Here's the drawing with two shaded views (mm, measured from the low corner). I have some questions. A direction names the side the tool comes from. Round coordinates to 2 decimals unless told otherwise and drop trailing zeros. Loops run counter-clockwise (first coordinate to the right, second up) from the corner with the lowest first, then second, coordinate; pieces in that order, holes last.
(1) I want a section at D-D on y = 43. Write out the boundary of the cut face in (x, z).
(2) Thinking about a two-plate mould opening in X: for the marked faces 4, 5 and 6, which applies, released by +X, released by -X, zero draft, split by the parting line, or undercut?
(3) Will these pins go through, and if not, where does the flat tip stop? pin 1 Ø12 at (x, z) = (18.5, 36.5) entering from +Y; pin 2 Ø1 at (x, z) = (39, 53.5) entering from -Y; pin 3 Ø6 at (y, z) = (9, 31.5) entering from -X; pin 4 Ø1.5 at (x, z) = (18, 21) entering from +Y.
(4) I want a section at A-A on z = 24. Give the number of separate pieces and of enclosed holes in the cut face, plus the area to 3 significant figures.
(5) Which directions (+Z, -Z, +X, -X, +Y, -Y) give clear straight access to the entire face, cutting with the end or side of a thin tool? Please do the marked faces 1, 2 and 3.
(6) If I drill on line 1 along Y through (x, z) = (7, 36); line 2 along X through (y, z) = (25, 30); line 3 along X through (y, z) = (24, 23.5), over which ranges is the centre line in solid material (lowest first)?
(7) I want a section at C-C on x = 20. Write out the boundary of the cut face in (y, z).
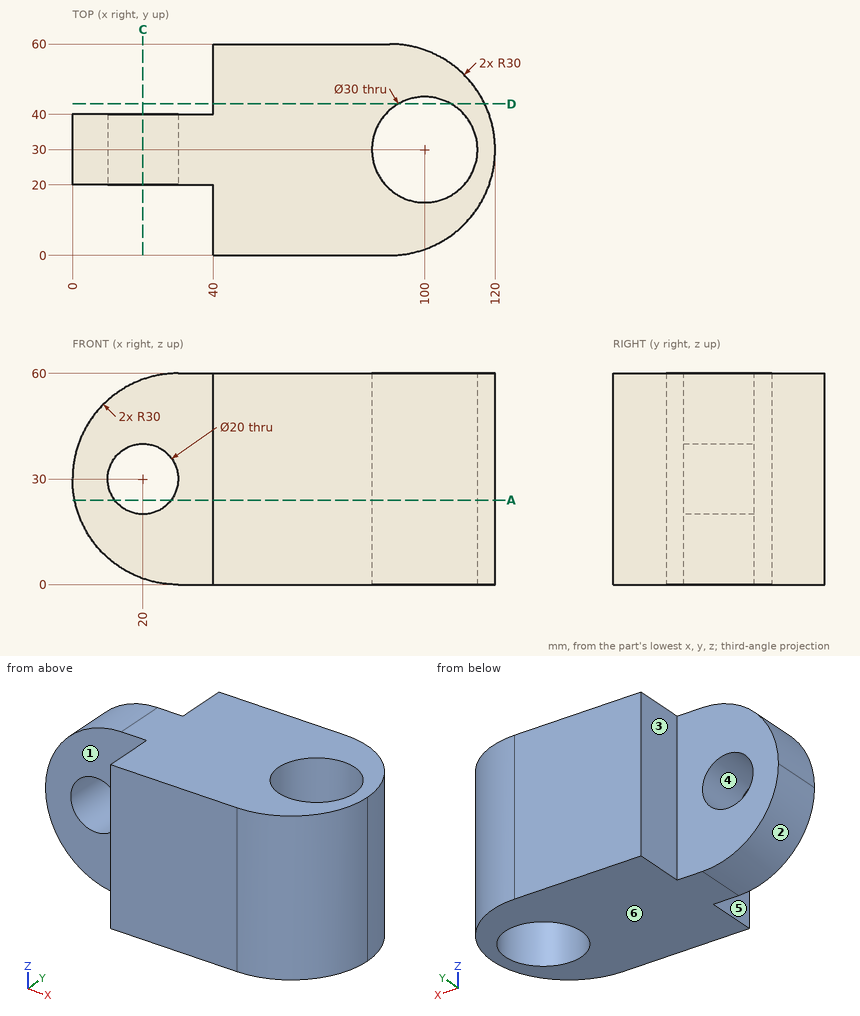
Filled sheet:
1. outline: (40, 0) - (92.52, 0) - (92.52, 60) - (40, 60) - close; (107.48, 0) - (117.04, 0) - (117.04, 60) - (107.48, 60) - close
2. face 4: undercut
2. face 5: released by -X
2. face 6: zero draft
3. pin 1: stops at y = 40
3. pin 2: stops at y = 20
3. pin 3: stops at x = 40
3. pin 4: passes through
4. separate pieces: 2
4. enclosed holes: 1
4. area: 4,170 mm2
5. face 1: +Z, -Z, -X, -Y
5. face 2: -Z, -X, +Y, -Y
5. face 3: +Z, -Z, -X, +Y
6. line 1: y = 20 to 40
6. line 2: x = 0 to 10, 30 to 85.86, 114.14 to 119.58
6. line 3: x = 0.71 to 12.4, 27.6 to 86.25, 113.75 to 119.39
7. outline: (20, 1.72) - (40, 1.72) - (40, 20) - (20, 20) - close; (20, 40) - (40, 40) - (40, 58.28) - (20, 58.28) - close
